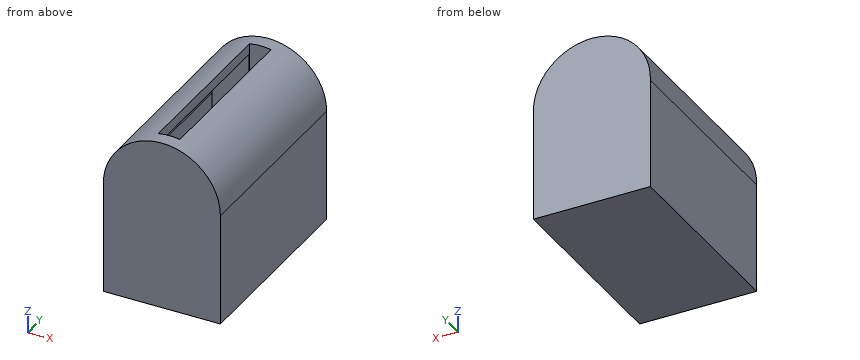
from build123d import *

# Parameters (mm, degrees)
F1_DEPTH = 49.022
F3_DEPTH = 41.656
F4_W     = 10.587335
F4_H     = 42.046845
F5_DEPTH = 108.712


with BuildPart() as f1:
    # F0 (on Front) → F1 (new body)
    with BuildSketch(Plane.XZ):
        with BuildLine():
            Line((-28.737051, 33.576977), (28.751377, 33.576977))
            ThreePointArc((28.751377, 33.576977), (-0.453801, 62.324772), (-28.737051, 32.669488))
            Line((-28.737051, 32.669488), (-28.737051, 33.576977))
        make_face()
        with BuildLine():
            ThreePointArc((-28.737051, 32.669488), (0.453801, 4.829181), (28.751377, 33.576977))
            Line((28.751377, 33.576977), (-28.737051, 33.576977))
            Line((-28.737051, 33.576977), (-28.737051, 32.669488))
        make_face()
        with BuildLine():
            Line((28.751377, -21.477165), (28.751377, 33.576977))
            ThreePointArc((28.751377, 33.576977), (0.453801, 4.829181), (-28.737051, 32.669488))
            Line((-28.737051, 32.669488), (-28.737051, -21.477165))
            Line((-28.737051, -21.477165), (28.751377, -21.477165))
        make_face()
    extrude(amount=F1_DEPTH)

    # F2 (on face) → F3 (cut)
    with BuildSketch(Plane(origin=(0, 0, 0), x_dir=(-1, 0, 0), z_dir=(0, 1, 0))):
        with BuildLine():
            ThreePointArc((23.594631, 31.736941), (23.648353, 32.656262), (23.66627, 33.576977))
            ThreePointArc((23.66627, 33.576977), (0, 57.243247), (-23.66627, 33.576977))
            Line((-23.66627, 33.576977), (23.594631, 33.576977))
            Line((23.594631, 33.576977), (23.594631, 31.736941))
        make_face()
        with BuildLine():
            Line((23.594631, 33.576977), (-23.66627, 33.576977))
            ThreePointArc((-23.66627, 33.576977), (-0.920715, 9.928623), (23.594631, 31.736941))
            Line((23.594631, 31.736941), (23.594631, 33.576977))
        make_face()
        with BuildLine():
            ThreePointArc((23.594631, 31.736941), (-0.920715, 9.928623), (-23.66627, 33.576977))
            Line((-23.66627, 33.576977), (-23.66627, -15.427259))
            Line((-23.66627, -15.427259), (23.594631, -15.427259))
            Line((23.594631, -15.427259), (23.594631, 31.736941))
        make_face()
    extrude(amount=-F3_DEPTH, mode=Mode.SUBTRACT)

    # F4 (on Top) → F5 (cut)
    with BuildSketch(Plane.XY):
        with Locations((-0.151248, -21.023422)):
            Rectangle(F4_W, F4_H)
    extrude(amount=F5_DEPTH, mode=Mode.SUBTRACT)

    # F6: F1 across plane


with BuildPart() as f1_1:
    add(f1.part)
    add(f1.part.mirror(Plane.XZ))


solid = f1_1.part
Verification items for the finished model (mm, model axes). Round coordinates to 2 decimals unless told otherwise and drop trailing zeros. Order: outer loops, then holes, each group sorted by start corner. A loop starts at its lowest first (then second) coordinate and runs counter-clockwise, first axis right, second up.
1. Thickness scan on L1, parallel to Y at x = 17.5, z = 43; L2, parallel to Y at x = 3, z = 33; L3, parallel to X at y = 41, z = 8. Record the ranges inside material, lowest first.
Final values:
L1: y = -49.02 to -41.66, 41.66 to 49.02
L2: y = -49.02 to -42.05, 42.05 to 49.02
L3: x = -28.74 to -23.59, 23.67 to 28.75
2. Section check C-C on y = 36.5. Record the cut outline in (x, z).
Final values:
outline: (-28.74, -21.48) - (28.75, -21.48) - (28.75, 33.58) arc R28.75 ccw to (5.14, 61.86) - (5.14, 56.68) arc R23.67 cw to (23.67, 33.58) - (23.67, -15.43) - (-23.59, -15.43) - (-23.59, 31.74) arc R23.67 cw to (-23.67, 33.58) arc R23.67 cw to (-5.44, 56.61) - (-5.44, 61.81) arc R28.75 ccw to (-28.74, 32.67) - close
3. Go/stop test with flat-tipped pins: P1, Ø2, axis at x = -22, y = 10.5, coming from the +Z side; P2, Ø1, axis at x = -12.5, y = 31, coming from the +Z side. Record where each tip stops, or that it passes through.
Final values:
P1: stops at z = 53.21
P2: stops at z = 59.7
4. Section check D-D on x = 0. Record the cut outline in (y, z).
Final values:
outline: (-49.02, -21.48) - (49.02, -21.48) - (49.02, 62.33) - (42.05, 62.33) - (42.05, 0) - (41.66, 0) - (41.66, -15.43) - (-41.66, -15.43) - (-41.66, 0) - (-42.05, 0) - (-42.05, 62.33) - (-49.02, 62.33) - close
5. Section check A-A on z = 7.5. Record the cut outline in (x, y), then the cut area to 3 significant figures.
Final values:
outline: (-28.74, -49.02) - (28.75, -49.02) - (28.75, 49.02) - (-28.74, 49.02) - close; hole (-23.59, -41.66) - (-5.44, -41.66) - (-5.44, -42.05) - (5.14, -42.05) - (5.14, -41.66) - (23.67, -41.66) - (23.67, 41.66) - (5.14, 41.66) - (5.14, 42.05) - (-5.44, 42.05) - (-5.44, 41.66) - (-23.59, 41.66) - close
area: 1,690 mm2
6. Section check B-B on x = -9. Record the cut outline in (y, z), then the cut area to 3 significant figures.
Final values:
outline: (-49.02, -21.48) - (49.02, -21.48) - (49.02, 60.88) - (-49.02, 60.88) - close; hole (-41.66, -15.43) - (41.66, -15.43) - (41.66, 55.47) - (-41.66, 55.47) - close
area: 2,170 mm2
